from build123d import *

# Parameters (mm, degrees)
EXTRUDE_1_DEPTH  = 50
EXTRUDE_START    = -50
EXTRUDE_3_DEPTH  = 70
SKETCH_5_W       = 13.017082793
SKETCH_5_H       = 9
EXTRUDE_4_DEPTH  = 18.5
SKETCH_6_W       = 13.017082793
SKETCH_6_H       = 9
EXTRUDE_5_DEPTH  = 16
EXTRUDE_6_DEPTH  = 50
SKETCH_9_W       = 5
SKETCH_9_H       = 6.401843996
EXTRUDE_7_DEPTH  = 10
SKETCH_10_W      = 5
SKETCH_10_H      = 6.401843997
EXTRUDE_8_DEPTH  = 10
SKETCH_11_R      = 2
EXTRUDE_9_DEPTH  = 30
SKETCH_15_R      = 2
EXTRUDE_10_DEPTH = 30
EXTRUDE_11_DEPTH = 5


with BuildPart() as part:
    # 草图1 → 凸台-拉伸1 (new body)
    with BuildSketch(Plane(origin=(0, 0, 0), x_dir=(1, 0, 0), z_dir=(0, 1, 0))):
        with BuildLine():
            Line((7.810249676, 50), (0, 50))
            Line((0, 50), (60, 0))
            Line((60, 0), (-0.663965605, -50.553304671))
            Line((-0.663965605, -50.553304671), (-0.663965605, -56.955148667))
            Line((-0.663965605, -56.955148667), (63.841106398, -3.200921998))
            ThreePointArc((63.841106398, -3.200921998), (64.979466032, 0.45267873), (63.200921998, 3.841106398))
            Line((63.200921998, 3.841106398), (7.810249676, 50))
        make_face()
    extrude(amount=EXTRUDE_1_DEPTH)

    # 草图4 → 凸台-拉伸3 (add)
    with BuildSketch(Plane(origin=(0, 50, 0), x_dir=(1, 0, 0), z_dir=(0, 1, 0)).offset(EXTRUDE_START)):
        Polygon((7.810249676, 50), (0, 50), (7.682212796, 43.598156003), (10.883134794, 47.439262401), align=None)
        Polygon((13.017082793, 50), (7.810249676, 50), (10.883134794, 47.439262401), align=None)
    extrude_3 = extrude(amount=EXTRUDE_3_DEPTH)

    # 草图5 → 凸台-拉伸4 (add)
    with BuildSketch(Plane(origin=(0, 0, -50), x_dir=(-1, 0, 0), z_dir=(0, 0, -1))):
        with Locations((-6.508541397, 65.5)):
            Rectangle(SKETCH_5_W, SKETCH_5_H)
    extrude_4 = extrude(amount=EXTRUDE_4_DEPTH)

    # 草图6 → 凸台-拉伸5 (add)
    with BuildSketch(Plane.XZ.offset(-61)):
        with Locations((6.508541397, -64)):
            Rectangle(SKETCH_6_W, SKETCH_6_H)
    extrude_5 = extrude(amount=EXTRUDE_5_DEPTH)

    # 镜向4: 凸台-拉伸3, 凸台-拉伸4, 凸台-拉伸5 across plane
    add(extrude_3.mirror(Plane(origin=(0, 25, 0), x_dir=(0, 0, 1), z_dir=(0, -1, 0))))
    add(extrude_4.mirror(Plane(origin=(0, 25, 0), x_dir=(0, 0, 1), z_dir=(0, -1, 0))))
    add(extrude_5.mirror(Plane(origin=(0, 25, 0), x_dir=(0, 0, 1), z_dir=(0, -1, 0))))

    # 草图8 → 凸台-拉伸6 (add)
    with BuildSketch(Plane(origin=(0, 50, 0), x_dir=(1, 0, 0), z_dir=(0, 1, 0))):
        Polygon((7.682212796, 43.598156003), (-0.663965605, 43.598156003), (-0.663965605, 50), (0, 50), align=None)
    extrude(amount=-EXTRUDE_6_DEPTH)

    # 草图9 → 凸台-拉伸7 (add)
    with BuildSketch(Plane.XZ):
        with Locations((-3.163965605, 53.754226669)):
            Rectangle(SKETCH_9_W, SKETCH_9_H)
        with BuildLine():
            Line((-5.663965605, 56.955148667), (-5.663965605, 50.553304671))
            ThreePointArc((-5.663965605, 50.553304671), (-8.864887603, 53.754226669), (-5.663965605, 56.955148667))
        make_face()
    extrude_7 = extrude(amount=-EXTRUDE_7_DEPTH)

    # 草图10 → 凸台-拉伸8 (add)
    with BuildSketch(Plane.XZ):
        with Locations((-3.163965605, -46.799078001)):
            Rectangle(SKETCH_10_W, SKETCH_10_H)
        with BuildLine():
            Line((-5.663965605, -43.598156003), (-5.663965605, -50))
            ThreePointArc((-5.663965605, -50), (-8.864887603, -46.799078002), (-5.663965605, -43.598156003))
        make_face()
    extrude_8 = extrude(amount=-EXTRUDE_8_DEPTH)

    # 镜向5: 凸台-拉伸7, 凸台-拉伸8 across plane
    add(extrude_7.mirror(Plane(origin=(0, 25, 0), x_dir=(0, 0, 1), z_dir=(0, -1, 0))))
    add(extrude_8.mirror(Plane(origin=(0, 25, 0), x_dir=(0, 0, 1), z_dir=(0, -1, 0))))

    # 草图11 → 凸台-拉伸9 (add)
    with BuildSketch(Plane.XZ.offset(-40)):
        with Locations((-5.663965605, 53.754226669)):
            Circle(SKETCH_11_R)
    extrude(amount=EXTRUDE_9_DEPTH)

    # 草图14 → 旋转1 (revolve)
    with BuildSketch(Plane(origin=(0, 0, 53.754226669), x_dir=(-1, 0, 0), z_dir=(0, 0, -1))):
        Polygon((7.663965605, 12.5), (7.663965605, 10), (8.864887603, 10), align=None)
        Polygon((7.663965605, 12.5), (8.864887603, 10), (7.663965605, 10), align=None)
    revolve_1 = revolve(axis=Axis((-5.663965605, 10, 53.754226669), (0, 1, 0)))

    # 镜向6: 旋转1 across plane
    add(revolve_1.mirror(Plane(origin=(0, 25, 0), x_dir=(0, 0, 1), z_dir=(0, -1, 0))))

    # 草图15 → 凸台-拉伸10 (add)
    with BuildSketch(Plane(origin=(0, 10, 0), x_dir=(1, 0, 0), z_dir=(0, 1, 0))):
        with Locations((-5.663965605, 46.799078002)):
            Circle(SKETCH_15_R)
    extrude(amount=EXTRUDE_10_DEPTH)

    # 草图17 → 旋转2 (revolve)
    with BuildSketch(Plane.XY.offset(-46.799078002)):
        Polygon((-7.663965605, 10), (-7.663965605, 12.5), (-8.864887603, 10), align=None)
    revolve_2 = revolve(axis=Axis((-5.663965605, 40, -46.799078002), (0, -1, 0)))

    # 镜向7: 旋转2 across plane
    add(revolve_2.mirror(Plane(origin=(0, 25, 0), x_dir=(0, 0, 1), z_dir=(0, -1, 0))))

    # 草图18 → 凸台-拉伸11 (add)
    with BuildSketch(Plane(origin=(24.590163934, 0, -29.508196721), x_dir=(0.76822128, 0, 0.6401844), z_dir=(-0.6401844, 0, 0.76822128))):
        Polygon((-22.009219983, 50), (-22.009219983, 70), (-2.009219983, 50), align=None)
    extrude_11 = extrude(amount=-EXTRUDE_11_DEPTH)

    # 镜向8: 凸台-拉伸11 across plane
    add(extrude_11.mirror(Plane(origin=(0, 25, 0), x_dir=(0, 0, 1), z_dir=(0, -1, 0))))


solid = part.part
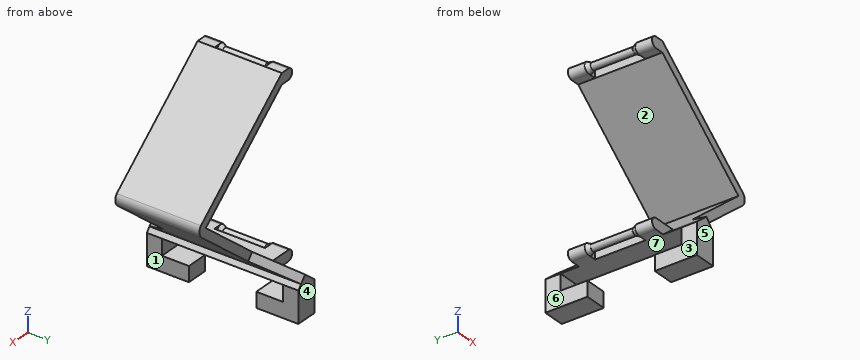
Input: part model. Units: mm. Frame: model coordinates. Face numbers are marked on the shaded views. A direction names the side the tool comes from. Round coordinates to 2 decimals unless told otherwise and drop trailing zeros. Write each loop counter-clockwise with the first axis right and the second up, starting at its lowest first coordinate (ties: lowest second). Pieces come first, ordered by that corner, then holes.
1) Ray query, L1, parallel to Y at x = 31, z = -24.5; L2, parallel to X at y = -13, z = -60; L3, parallel to Z at x = 7.5, y = 59.5. Return the intervals inside material, ascending.
2) Reachability of the marked faces 1, 2 and 3 from +Z, -Z, +X, -X, +Y, -Y: full face, straight path, thin tool, end or side. Return the list, or none.
3) Cut plane B-B (x = 29). Return the cut outline in (y, z).
4) Cut plane A-A (y = 7). Return the cut outline in (x, z), then the cut area to 3 significant figures.
5) Draft query along Y for the marked faces 4, 5, 6 and 7. Return one class per face: pulls with the +Y half, pulls with the -Y half, needs draft (parallel to the pull), parting line crosses it, or undercut.
6) Contact query for flat-ended pins moving along their axis: P1, Ø9, axis at y = 53.5, z = -55.5, coming from the +X side; P2, Ø5, axis at x = -2.5, z = -47.5, coming from the +Y side; P3, Ø4, axis at x = -2.5, y = 4, coming from the -Z side; P4, Ø12, axis at y = 58.5, z = -24, coming from the -X side. Output: stop coordinate, or through.
7) Cut plane D-D (y = 35). Return the cut outline in (x, z).
8) Cut plane C-C (y = -8). Return the cut outline in (x, z).
Geometry says:
1. L1: y = 0 to 50
1. L2: x = 0 to 13.02
1. L3: z = -68.5 to -59.5, -50 to -43.75
2. face 1: -Z, +X, +Y, -Y
2. face 2: -X, +Y, -Y
2. face 3: -Z, -X, +Y, -Y
3. outline: (0, -32.34) - (50, -32.34) - (50, -25.83) - (0, -25.83) - close; (0, 25.83) - (50, 25.83) - (50, 32.24) - (0, 32.24) - close
4. outline: (-5.66, -50) - (13.02, -50) - (10.88, -47.44) - (63.2, -3.84) arc R5 ccw to (63.84, 3.2) - (-0.66, 56.96) - (-5.66, 56.96) arc R3.2 ccw to (-5.66, 50.55) - (-0.66, 50.55) - (60, 0) - (7.68, -43.6) - (-5.66, -43.6) arc R3.2 ccw to start
4. area: 928 mm2
5. face 4: pulls with the +Y half
5. face 5: pulls with the -Y half
5. face 6: needs draft
5. face 7: undercut
6. P1: stops at x = 13.02
6. P2: stops at y = 50
6. P3: stops at z = -50
6. P4: passes through
7. outline: circle Ø4 at (-5.66, -46.8); circle Ø4 at (-5.66, 53.75); (-0.66, -50) - (13.02, -50) - (10.88, -47.44) - (63.2, -3.84) arc R5 ccw to (63.84, 3.2) - (-0.66, 56.96) - (-0.66, 50.55) - (60, 0) - (7.68, -43.6) - (-0.66, -43.6) - close
8. outline: (0, -68.5) - (13.02, -68.5) - (13.02, -59.5) - (0, -59.5) - close; (0, -50) - (13.02, -50) - (10.88, -47.44) - (20.1, -39.76) - (16.9, -35.92) - close
